Verification items for the finished model (mm, model axes). Coordinates: 2 decimals unless noted, no trailing zeros. Order: outer loops, then holes, each group sorted by start corner. A loop starts at its lowest first (then second) coordinate and runs counter-clockwise, first axis right, second up. Notation, with made-up numbers: (-39.75, -9) - (-1.75, -9) arc R18 cw to (-1.75, 4) - close; hole circle Ø4 at (88.5, 60.5). An arc over 180 degrees is marked (long way). Answer as CSV lines item,"result". Start each with the question number.
1. Section check C-C (z = 0.7). Count the separate pieces of the cut face and the enclosed holes in it, and give its area (3 significant figures).
2. Material ranges on L1, parallel to Y at x = 4, z = 0.35; L2, parallel to Y at x = 4.75, z = 0.85; L3, parallel to X at y = 3.5, z = 0.75, recorded low to high. Write a range as [from, to].
3. Section check B-B (x = 4). Record the cut outline in (y, z).
4. Go/stop test with a flat-tipped pin: pin 1 (1.7 mm diameter, centred on x = 20.77, y = 28, fed in from +Z). Record where the tip stops, or that it passes through.
5. Section check A-A (y = 34). Record the cut outline in (x, z).
6. Section check D-D (y = 9). Record the cut outline in (x, z).
7. Mould release check, pull along X, two halves, no side actions. Record for faces 1 (the flat face through (0, 25, 1)), 2 (the flat face through (13, 25, 1.3)), 3 (the cylindrical face through (22.106, 39.445, 0.641)), 4 (the flat face through (25, 25, 1)): pulls with the +X half, pulls with the -X half, needs draft (parallel to the pull), parting line crosses it, or undercut.
from build123d import *

# Parameters (mm, degrees)
SKETCH1_R           = 1.6
SKETCH1_R_2         = 1.45
BOSS_EXTRUDE1_DEPTH = 1.3
FILLET1_R           = 2


with BuildPart() as part:
    # Sketch1 → Boss-Extrude1 (new body)
    with BuildSketch(Plane.XY):
        Polygon((12, 50), (25, 48.75), (25, 1.25), (12, 0), (0, 0), (0, 50), align=None)
        with Locations((4, 46.213205)):
            Circle(SKETCH1_R, mode=Mode.SUBTRACT)
        with Locations((4, 3.786795)):
            Circle(SKETCH1_R, mode=Mode.SUBTRACT)
        with Locations((20.766795, 46)):
            Circle(SKETCH1_R_2, mode=Mode.SUBTRACT)
        with Locations((20.766795, 4)):
            Circle(SKETCH1_R_2, mode=Mode.SUBTRACT)
        with Locations((20.766795, 40)):
            Circle(SKETCH1_R_2, mode=Mode.SUBTRACT)
        with Locations((20.766795, 34)):
            Circle(SKETCH1_R_2, mode=Mode.SUBTRACT)
        with Locations((20.766795, 28)):
            Circle(SKETCH1_R_2, mode=Mode.SUBTRACT)
        with Locations((20.766795, 22)):
            Circle(SKETCH1_R_2, mode=Mode.SUBTRACT)
        with Locations((20.766795, 16)):
            Circle(SKETCH1_R_2, mode=Mode.SUBTRACT)
        with Locations((20.766795, 10)):
            Circle(SKETCH1_R_2, mode=Mode.SUBTRACT)
    extrude(amount=BOSS_EXTRUDE1_DEPTH)

    # Fillet1
    fillet1_edges = [part.edges().sort_by_distance(p)[0] for p in [
        (0, 50, 0.65),
        (25, 48.75, 0.65),
        (25, 1.25, 0.65),
        (0, 0, 0.65),
    ]]
    fillet(fillet1_edges, radius=FILLET1_R)


solid = part.part
Evaluation:
1,separate pieces,"1"
1,enclosed holes,"10"
1,area,"1,160 mm²"
2,L1,"y = [0, 2.19], [5.39, 44.61], [47.81, 50]"
2,L2,"y = [0, 2.37], [5.2, 44.8], [47.63, 50]"
2,L3,"x = [0, 2.43], [5.57, 19.41], [22.13, 25]"
3,outline,"(0, 0) - (2.19, 0) - (2.19, 1.3) - (0, 1.3) - close; (5.39, 0) - (44.61, 0) - (44.61, 1.3) - (5.39, 1.3) - close; (47.81, 0) - (50, 0) - (50, 1.3) - (47.81, 1.3) - close"
4,pin 1,"passes through"
5,outline,"(0, 0) - (19.32, 0) - (19.32, 1.3) - (0, 1.3) - close; (22.22, 0) - (25, 0) - (25, 1.3) - (22.22, 1.3) - close"
6,outline,"(0, 0) - (19.72, 0) - (19.72, 1.3) - (0, 1.3) - close; (21.82, 0) - (25, 0) - (25, 1.3) - (21.82, 1.3) - close"
7,face 1,"pulls with the -X half"
7,face 2,"needs draft"
7,face 3,"undercut"
7,face 4,"pulls with the +X half"
